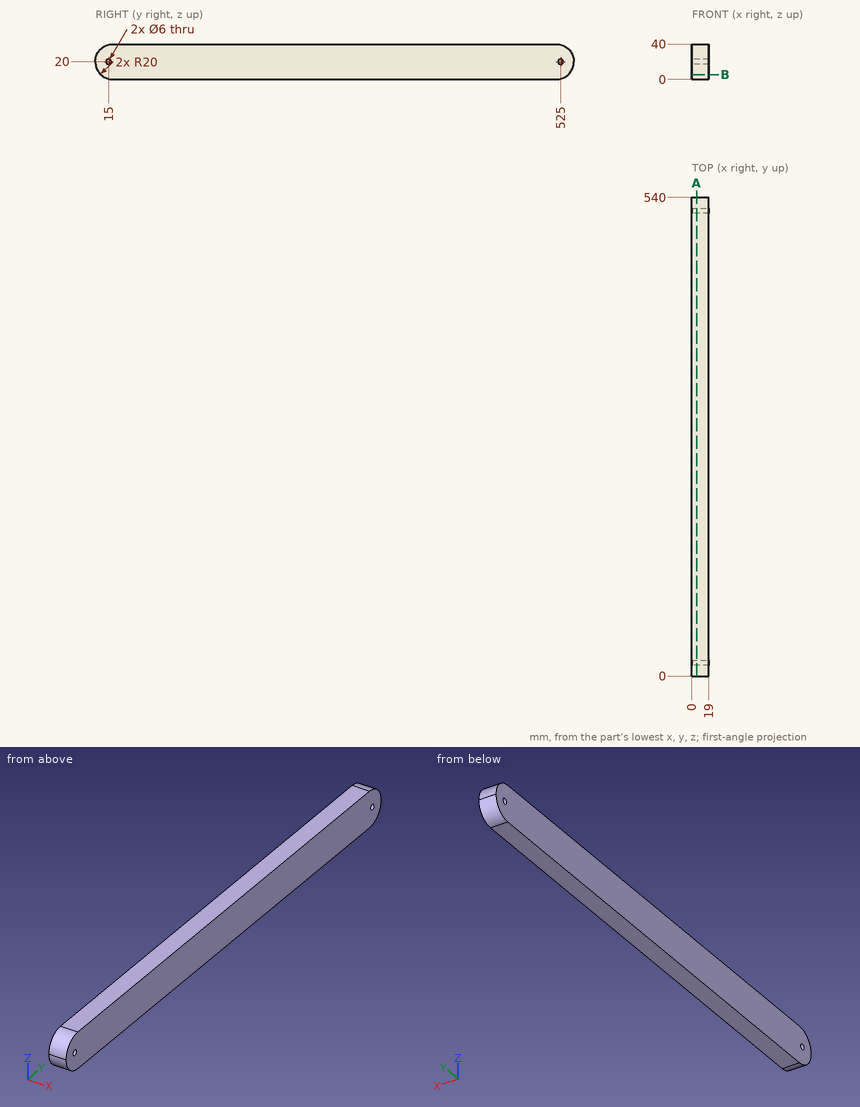
Here's the drawing with two shaded views (mm, measured from the low corner). I have some questions. Give positions to 0.01 mm unless a question says otherwise; leave off trailing zeros. Loops run counter-clockwise (first coordinate to the right, second up) from the corner with the lowest first, then second, coordinate; pieces in that order, holes last. Notation, with made-up numbers: M -36,37.5 L 18,37.5 A18 ccw 18,43.5 Z; hole C 16.25,-35.5 d1. An arc over 180 degrees is marked long. Answer in a Markdown table with one row per item.
1. Suppose I cut it at B-B on z = 5.5. Write out the boundary of the cut face in (x, y) (3 decimals), plus the area to 3 significant figures.
Taken from the geometry:
| item | result |
|---|---|
| outline | M 0,6.225 L 19,6.225 L 19,533.775 L 0,533.775 Z |
| area | 10,000 mm² |
2. If I drill on line 1 along Y through (x, z) = (5.5, 21) (3 decimals); line 2 along Z through (x, y) = (4, 525); line 3 along Y through (x, z) = (14.75, 36.5), over which ranges is the centre line in solid material (lowest first)?
Taken from the geometry:
| item | result |
|---|---|
| line 1 | y = 0.025 to 12.172, 17.828 to 522.172, 527.828 to 539.975 |
| line 2 | z = 0.64 to 17, 23 to 39.36 |
| line 3 | y = 8.7 to 531.3 |
3. For pin 1 Ø5 at (x, z) = (9, 7.5) entering from +Y; pin 2 Ø5 at (x, z) = (6, 13) entering from -Y, each with a flat end and sliding along its axis, tell me the tip position at first contact or that it passes through.
Taken from the geometry:
| item | result |
|---|---|
| pin 1 | stops at y = 537.32 |
| pin 2 | stops at y = 0.51 |
4. Suppose I cut it at A-A on x = 5.25. Count the separate pieces of the cut face and the enclosed holes in it, plus the area to 3 significant figures.
Taken from the geometry:
| item | result |
|---|---|
| separate pieces | 1 |
| enclosed holes | 2 |
| area | 21,200 mm² |
